```python
from build123d import *

# Parameters (mm, degrees)
SKETCH3_R          = 6.35
CUT_EXTRUDE1_DEPTH = 81.161047897
FILLET1_R          = 6.35


with BuildPart() as part:
    # Sketch2 → Revolve1 (revolve)
    with BuildSketch(Plane.XY, mode=Mode.PRIVATE) as revolve1_sk:
        Polygon((45.72, 17.272), (20.32, 17.272), (20.32, 23.622), (10.16, 23.622), (10.16, 50.8), (7.62, 50.8), (7.62, 48.26), (0, 48.26), (0, 50.8), (-2.54, 50.8), (-2.54, 12.7), (0, 12.7), (0, 0), (45.72, 0), align=None)
    revolve(revolve1_sk.sketch.rotate(Axis((-1001.184765233, 0, 0), (1, 0, 0)), 90), axis=Axis((-1001.184765233, 0, 0), (1, 0, 0)))

    # Sketch3 → Cut-Extrude1 (cut, through all)
    with BuildSketch(Plane(origin=(10.16, 0, 0), x_dir=(0, 0, -1), z_dir=(1, 0, 0))):
        with Locations((26.312150435, 26.312150435)):
            Circle(SKETCH3_R)
        with Locations((0, 37.211)):
            Circle(SKETCH3_R)
        with Locations((37.211, 0)):
            Circle(SKETCH3_R)
        with Locations((26.312150435, -26.312150435)):
            Circle(SKETCH3_R)
        with Locations((0, -37.211)):
            Circle(SKETCH3_R)
        with Locations((-26.312150435, -26.312150435)):
            Circle(SKETCH3_R)
        with Locations((-37.211, 0)):
            Circle(SKETCH3_R)
        with Locations((-26.312150435, 26.312150435)):
            Circle(SKETCH3_R)
    extrude(amount=-CUT_EXTRUDE1_DEPTH, mode=Mode.SUBTRACT)

    # Fillet1
    fillet1_edges = [part.edges().sort_by_distance(p)[0] for p in [
        (20.32, 0, -17.272),
    ]]
    fillet(fillet1_edges, radius=FILLET1_R - 0.0001)  # a hair under: the kernel refuses the full size


solid = part.part
```
Part model, mm, in its own coordinate system. A direction names the side the tool comes from. Round coordinates to 2 decimals unless told otherwise and drop trailing zeros. Write each loop counter-clockwise with the first axis right and the second up, starting at its lowest first coordinate (ties: lowest second). Pieces come first, ordered by that corner, then holes.
Item 1: Drop flat-ended pins along their axis: pin 1 Ø14.5 at (y, z) = (0, -37.211) entering from +X; pin 2 Ø10 at (y, z) = (-26.31, -26.31) entering from +X; pin 3 Ø2 at (x, z) = (10, -2) entering from -Y; pin 4 Ø4 at (x, y) = (40, -16) entering from +Z. Give the stop position or say it passes through.
Results:
pin 1: stops at x = 10.16
pin 2: passes through
pin 3: stops at y = -50.79
pin 4: stops at z = 10.12
Item 2: Cut at D-D, the plane y = -34.5. Give the cut face in (x, z), plus the area to 3 significant figures.
Results:
outline: (-2.54, -37.29) - (0, -37.29) - (0, -33.75) - (7.62, -33.75) - (7.62, -37.29) - (10.16, -37.29) - (10.16, -5.74) - (-2.54, -5.74) - close; (-2.54, 5.74) - (10.16, 5.74) - (10.16, 37.29) - (7.62, 37.29) - (7.62, 33.75) - (0, 33.75) - (0, 37.29) - (-2.54, 37.29) - close
area: 747 mm2
Item 3: Probe L1, parallel to X at y = 10, z = 44.5; L2, parallel to X at y = 6, z = -8.5; L3, parallel to Y at x = 8, z = -39. List the from-to ranges inside material, lowest first.
Results:
L1: x = -2.54 to 10.16
L2: x = 0 to 45.72
L3: y = -32.55 to -6.09, 6.09 to 32.55
Item 4: Cut at A-A, the plane y = 0. Count the separate pieces of the cut face and the enclosed holes in it, plus the area to 3 significant figures.
Results:
separate pieces: 3
enclosed holes: 0
area: 2,240 mm2
Item 5: Two-plate mould, pull along Y, no slides. Class faces 1 (the cylindrical face through (3.899, -31.946, -29.242)), 2 (the flat face through (45.72, 0, 0)), 3 (the cylindrical face through (8.872, 30.911, -40.313)): +Y half, -Y half, draft (parallel to the pull), parting line (faces both ways), or undercut.
Results:
face 1: undercut
face 2: draft
face 3: parting line
Item 6: Cut at C-C, the plane z = 41. Give the cut face in (x, y).
Results:
outline: (-2.54, -29.99) - (0, -29.99) - (0, -25.46) - (7.62, -25.46) - (7.62, -29.99) - (10.16, -29.99) - (10.16, -5.1) - (-2.54, -5.1) - close; (-2.54, 5.1) - (10.16, 5.1) - (10.16, 29.99) - (7.62, 29.99) - (7.62, 25.46) - (0, 25.46) - (0, 29.99) - (-2.54, 29.99) - close
Item 7: Which spindle directions (+Z, -Z, +X, -X, +Y, -Y) get a long thin tool onto all of the face, cutting with end or side? Do faces 4 (the cylindrical face through (3.9, 23.88, -32.18)), 5 (the flat face through (0, 0, 0)), 6 (the cylindrical face through (15.17, 14.37, -18.75)), 7 (the cylindrical face through (3.76, -14.5, 46.03)). Say none if no direction does.
Results:
face 4: +X, -X
face 5: -X
face 6: +X
face 7: none
